```python
from build123d import *

# Parameters (mm, degrees)
SKETCH1_R           = 1.5
SKETCH1_R_2         = 2
BOSS_EXTRUDE1_DEPTH = 1.5


with BuildPart() as part:
    # Sketch1 → Boss-Extrude1 (new, symmetric)
    with BuildSketch(Plane(origin=(0, 0, 0), x_dir=(1, 0, 0), z_dir=(0, 1, 0))):
        with BuildLine():
            Line((-17.5, 4), (-11.5, 4))
            ThreePointArc((-11.5, 4), (-9.787250471, 2.753376432), (-7.807350165, 2))
            Line((-7.807350165, 2), (6.326731681, 2))
            ThreePointArc((6.326731681, 2), (8.998056486, 2.061872567), (11.5, 3))
            Line((11.5, 3), (17.5, 3))
            ThreePointArc((17.5, 3), (20.5, 0), (17.5, -3))
            Line((17.5, -3), (11.5, -3))
            ThreePointArc((11.5, -3), (8.998056486, -2.061872567), (6.326731681, -2))
            Line((6.326731681, -2), (-7.807350165, -2))
            ThreePointArc((-7.807350165, -2), (-9.787250471, -2.753376432), (-11.5, -4))
            Line((-11.5, -4), (-17.5, -4))
            ThreePointArc((-17.5, -4), (-21.5, 0), (-17.5, 4))
        make_face()
        with Locations(Location((17.5, 0, 0), (0, 0, 270))):
            Circle(SKETCH1_R, mode=Mode.SUBTRACT)
        with Locations(Location((-17.5, 0, 0), (0, 0, 270))):
            Circle(SKETCH1_R_2, mode=Mode.SUBTRACT)
    extrude(amount=BOSS_EXTRUDE1_DEPTH, both=True)


solid = part.part
```
Source: CAD feature listing. Evaluate the final solid. Frame: model axes, mm. A direction names the side the tool comes from. Round coordinates to 2 decimals unless told otherwise and drop trailing zeros. Loops run counter-clockwise (first coordinate to the right, second up) from the corner with the lowest first, then second, coordinate; pieces in that order, holes last. Notation, with made-up numbers: M -1.5,7.5 L 54.5,7.5 A29 ccw 54.5,42.5 Z; hole C -38,44 d10. An arc over 180 degrees is marked long. Use a Markdown table: item, result. Add a question column.
1. Set-up query: faces 4 (the flat face through (14, 0, -3)), 5 (the flat face through (15, 0, 3)), 6 (the flat face through (-1, 0, 2)). Return all of +Z, -Z, +X, -X, +Y, -Y with unobstructed straight access to the full face (end or side cutting, diameter ignored); none if empty.
2. Pull-direction query (Z, two-part tool) for faces 1 (the cylindrical face through (-9.813, 0.021, -2.768)), 2 (the cylindrical face through (-15.517, -0.021, -0.26)), 3 (the cylindrical face through (-9.76, 0.02, 2.74)); classes: +Z half, -Z half, draft (parallel to the pull), parting line (faces both ways), or undercut.
3. Cut plane C-C, the plane x = -1. Output: boundary loops of the cut face in (y, z).
4. Cut plane D-D, the plane x = 15.5. Output: boundary loops of the cut face in (y, z).
5. Ray query, line 1 along X through (y, z) = (0.3, 0); line 2 along X through (y, z) = (-0.35, -1); line 3 along Z through (x, y) = (-6, 1.2). Return the intervals inside material, ascending. Write a range as [from, to].
6. Cut plane B-B, the plane y = -0.7. Output: boundary loops of the cut face in (x, z).
7. Cut plane A-A, the plane z = 0. Output: boundary loops of the cut face in (x, y), and give its area (3 significant figures).
8. Contact query for flat-ended pins moving along their axis: pin 1 (0.9 mm diameter, centred on x = 15.5, y = 0.5, fed in from -Z); pin 2 (2.5 mm diameter, centred on x = 17.5, z = 0, fed in from +Y); pin 3 (1.5 mm diameter, centred on x = 14, y = -0.5, fed in from +Z); pin 4 (1.5 mm diameter, centred on y = 1, z = 2, fed in from -X). Output: stop coordinate, or through.
Solution:
| question | item | result |
|---|---|---|
| 1 | face 4 | -Z, +X, +Y, -Y |
| 1 | face 5 | +Z, +X, +Y, -Y |
| 1 | face 6 | +Z, +Y, -Y |
| 2 | face 1 | -Z half |
| 2 | face 2 | undercut |
| 2 | face 3 | +Z half |
| 3 | outline | M -1.5,-2 L 1.5,-2 L 1.5,2 L -1.5,2 Z |
| 4 | outline | M -1.5,-3 L 1.5,-3 L 1.5,3 L -1.5,3 Z |
| 5 | line 1 | x = [-21.5, -19.5], [-15.5, 16], [19, 20.5] |
| 5 | line 2 | x = [-21.37, -19.23], [-15.77, 16.38], [18.62, 20.33] |
| 5 | line 3 | z = [-2, 2] |
| 6 | outline | M -17.5,-4 L -11.5,-4 A8 cw -7.81,-2 L 6.33,-2 A8 cw 11.5,-3 L 17.5,-3 A3 ccw 17.5,3 L 11.5,3 A8 cw 6.33,2 L -7.81,2 A8 cw -11.5,4 L -17.5,4 A4 ccw Z; hole C -17.5,0 d4; hole C 17.5,0 d3 |
| 7 | outline | M -21.5,-1.5 L -19.5,-1.5 L -19.5,1.5 L -21.5,1.5 Z; M -15.5,-1.5 L 16,-1.5 L 16,1.5 L -15.5,1.5 Z; M 19,-1.5 L 20.5,-1.5 L 20.5,1.5 L 19,1.5 Z |
| 7 | area | 105 mm2 |
| 8 | pin 1 | stops at z = -3 |
| 8 | pin 2 | passes through |
| 8 | pin 3 | stops at z = 3 |
| 8 | pin 4 | stops at x = -21.3 |
